Check sheet for the modelled part. Datum: model origin and axes. Units: mm. Face numbers are marked on the shaded views. A direction names the side the tool comes from. Round coordinates to 2 decimals unless told otherwise and drop trailing zeros. Order: outer loops, then holes, each group sorted by start corner. A loop starts at its lowest first (then second) coordinate and runs counter-clockwise, first axis right, second up.
(1) Thickness scan on probe 1 along X at (y, z) = (-3, 4); probe 2 along Y at (x, z) = (25.5, 3); probe 3 along Z at (x, y) = (14, -14). Record the ranges inside material, lowest first.
(2) Sectioned sample at D-D, the plane y = 5. Enter the section's corners in (x, z).
(3) Tool access check on the marked faces 1, 2 and 3. Record the directions out of +Z, -Z, +X, -X, +Y, -Y that give a thin tool (end or side, any length) a straight path to the whole face; none if there is none.
(4) Depth check by flat-ended pin: pin 1 (1.8 mm diameter, centred on y = -2.5, z = 2.5, fed in from +X); pin 2 (8 mm diameter, centred on x = 2.5, y = -4.5, fed in from +Z). Enter the tip coordinate at first touch or a pass-through.
(5) Sectioned sample at A-A, the plane y = -5. Enter the section's corners in (x, z), and give its area (3 significant figures).
(6) Sectioned sample at C-C, the plane z = 5.3. Enter the section's corners in (x, y).
(7) Sectioned sample at B-B, the plane x = 10. Enter the section's corners in (y, z), and give its area (3 significant figures).
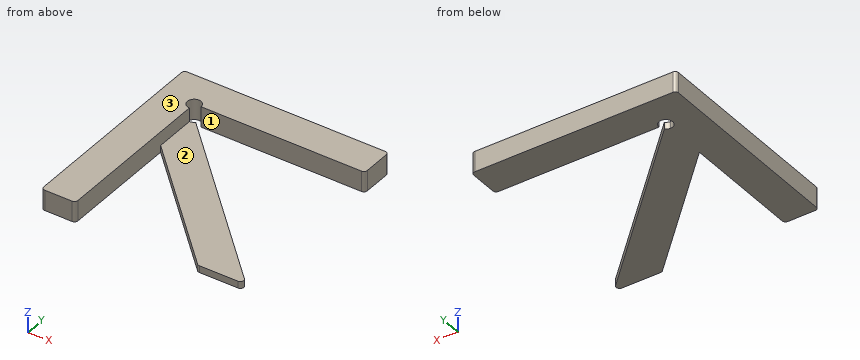
```python
from build123d import *

# Parameters (mm, degrees)
F1_DEPTH = 2
F2_DEPTH = 6
F3_R     = 1


with BuildPart() as f1:
    # F0 (on Top) → F1 (new body)
    with BuildSketch(Plane.XY):
        with BuildLine():
            ThreePointArc((0, -2), (-1.414214, 1.414214), (2, 0))
            Line((2, 0), (50, 0))
            Line((50, 0), (50, 10))
            Line((50, 10), (-10, 10))
            Line((-10, 10), (-10, -50))
            Line((-10, -50), (0, -50))
            Line((0, -50), (0, -14.142136))
            Line((0, -14.142136), (0, -2))
        make_face()
        with BuildLine():
            ThreePointArc((1.414214, -1.414214), (0.765367, -1.847759), (0, -2))
            Line((0, -2), (0, -14.142136))
            Line((0, -14.142136), (35.857864, -50))
            Line((35.857864, -50), (50, -50))
            Line((50, -50), (1.414214, -1.414214))
        make_face()
    extrude(amount=F1_DEPTH)

    # F0 (on Top) → F2 (join)
    with BuildSketch(Plane.XY):
        with BuildLine():
            ThreePointArc((0, -2), (-1.414214, 1.414214), (2, 0))
            Line((2, 0), (50, 0))
            Line((50, 0), (50, 10))
            Line((50, 10), (-10, 10))
            Line((-10, 10), (-10, -50))
            Line((-10, -50), (0, -50))
            Line((0, -50), (0, -14.142136))
            Line((0, -14.142136), (0, -2))
        make_face()
    extrude(amount=F2_DEPTH)

    # F3
    f3_edges = [f1.edges().sort_by_distance(p)[0] for p in [
        (-10, -50, 3),
        (0, -50, 3),
        (35.857864, -50, 1),
        (50, 0, 3),
        (50, 10, 3),
        (-10, 10, 3),
        (50, -50, 1),
    ]]
    fillet(f3_edges, radius=F3_R)


with BuildPart() as f1_1:
    # F4: moved
    add(f1.part.moved(Location((-10.68996, 11.8976, 0))))


solid = f1_1.part
```
Derived:
1. probe 1: x = -20.69 to -10.69
1. probe 2: y = 11.9 to 21.9
1. probe 3: z = 0 to 2
2. outline: (-20.69, 0) - (-3.79, 0) - (-3.79, 2) - (-10.69, 2) - (-10.69, 6) - (-20.69, 6) - close
3. face 1: +Z, -Z, +X
3. face 2: +Z, +X, -Y
3. face 3: +Z, +X, -X, +Y, -Y
4. pin 1: stops at x = 4.46
4. pin 2: stops at z = 2
5. outline: (-20.69, 0) - (-10.69, 0) - (-10.69, 6) - (-20.69, 6) - close; (-7.93, 0) - (6.21, 0) - (6.21, 2) - (-7.93, 2) - close
5. area: 88.3 mm2
6. outline: (-20.69, -37.1) arc R1 ccw to (-19.69, -38.1) - (-11.69, -38.1) arc R1 ccw to (-10.69, -37.1) - (-10.69, 9.9) arc R2 cw (long way) to (-8.69, 11.9) - (38.31, 11.9) arc R1 ccw to (39.31, 12.9) - (39.31, 20.9) arc R1 ccw to (38.31, 21.9) - (-19.69, 21.9) arc R1 ccw to (-20.69, 20.9) - close
7. outline: (-22.93, 0) - (-8.79, 0) - (-8.79, 2) - (-22.93, 2) - close; (11.9, 0) - (21.9, 0) - (21.9, 6) - (11.9, 6) - close
7. area: 88.3 mm2
